Autodesk Inventor part; units mm, degrees
ref_plane "YZ Plane" through (0, 0, 0) normal (1, 0, 0) x (0, 1, 0)
ref_plane "XZ Plane" through (0, 0, 0) normal (0, 1, 0) x (-1, 0, 0)
ref_plane "XY Plane" through (0, 0, 0) normal (0, 0, 1) x (1, 0, 0)
sketch "Sketch1" plane through (0, 0, 0) normal (0, 0, 1) x (1, 0, 0)
  line L0 (-50, 50) -> (50, 50)
  line L1 (50, 50) -> (50, -50)
  line L2 (50, -50) -> (-50, -50)
  line L3 (-50, -50) -> (-50, 50)
  line L4 (-92.7646, -8.503) -> (-89.7646, -8.503)
  line L5 (-89.7646, -8.503) -> (-89.7646, -11.753)
  line L6 (-89.7646, -11.753) -> (-92.7646, -11.753)
  line L7 (-92.7646, -11.753) -> (-92.7646, -8.503)
  line L8 (-92.7646, -21.6527) -> (-89.7646, -21.6527)
  line L9 (-89.7646, -21.6527) -> (-89.7646, -21.7527)
  line L10 (-89.7646, -21.7527) -> (-92.7646, -21.7527)
  line L11 (-92.7646, -21.7527) -> (-92.7646, -21.6527)
  line L12 (-50, 50) -> (-46.75, 50)
  line L13 (-46.75, 50) -> (-46.75, 36)
  line L14 (-46.75, 36) -> (-50, 36)
  line L15 (-50, 36) -> (-50, 50)
  line L16 (0, 50) -> (0, -50) construction
  line L17 (-50, 0) -> (50, 0) construction
  line L18 (50, 50) -> (46.75, 50)
  line L19 (46.75, 50) -> (46.75, 36)
  line L20 (46.75, 36) -> (50, 36)
  line L21 (50, 36) -> (50, 50)
  line L22 (-50, -50) -> (-46.75, -50)
  line L23 (-46.75, -50) -> (-46.75, -36)
  line L24 (-46.75, -36) -> (-50, -36)
  line L25 (-50, -36) -> (-50, -50)
  line L26 (46.75, -50) -> (46.75, -36)
  line L27 (46.75, -36) -> (50, -36)
  line L28 (50, -36) -> (50, -50)
  line L29 (50, -50) -> (46.75, -50)
  line L30 (-40, -50) -> (-10, -50)
  line L31 (-10, -50) -> (-10, -37)
  line L32 (-17, -30) -> (-33, -30)
  line L33 (-40, -37) -> (-40, -50)
  line L34 (40, -50) -> (10, -50)
  line L35 (10, -50) -> (10, -37)
  line L36 (17, -30) -> (33, -30)
  line L37 (40, -37) -> (40, -50)
  line L38 (-1.75, -50) -> (-5, -50)
  line L39 (-5, -50) -> (-5, -42)
  line L40 (-5, -42) -> (-1.75, -42)
  line L41 (-1.75, -42) -> (-1.75, -50)
  line L42 (1.75, -50) -> (5, -50)
  line L43 (5, -50) -> (5, -42)
  line L44 (5, -42) -> (1.75, -42)
  line L45 (1.75, -42) -> (1.75, -50)
  arc A0 (-33, -30) -> (-40, -37) centre (-33, -37) ccw
  arc A1 (-10, -37) -> (-17, -30) centre (-17, -37) ccw
  arc A2 (17, -30) -> (10, -37) centre (17, -37) ccw
  arc A3 (40, -37) -> (33, -30) centre (33, -37) ccw
  point P0 (0, 0)
  point P1 (-10, -30)
  point P2 (-40, -30)
  point P3 (10, -30)
  point P4 (40, -30)
  dimension "d0" = 100
  dimension "d2" = 100
  dimension "d3" = 3
  dimension "mat" = 3.25
  dimension "d5" = 3
  dimension "kerf" = 0.1
  dimension "d7" = 3.25
  dimension "d8" = 14
  dimension "d15" = 30
  dimension "d16" = 20
  dimension "d17" = 10
  dimension "d20" = 3.25
  dimension "d21" = 8
  dimension "d22" = 5
  dimension "d25" = 45
  dimension "d26" = 7
extrude "Extrusion2" add sketch "Sketch1" along normal blind 3.25 contours L0 L19 L20 L1 L27 L26 L2 L37 A3 L36 A2 L35 L43 L44 L45 L41 L40 L39 L31 A1 L32 A0 L33 L23 L24 L3 L14 L13 | L39 L40 L41 L2 | L45 L44 L43 L2
extrude "Extrusion3" cut sketch "Sketch1" along normal blind 3.25 contours L39 L40 L41 L2 | L45 L44 L43 L2
equation "\"d7\" = mat"
equation "\"d20\" = mat"
equation "\"d18\" = mat"
equation "\"d23\" = mat"
properties part number "body-back"
Read the model definition and answer for the solid it produces. Units are mm, in the model's axes. A direction names the side the tool comes from. Round coordinates to 2 decimals unless told otherwise and drop trailing zeros. Loops run counter-clockwise (first coordinate to the right, second up) from the corner with the lowest first, then second, coordinate; pieces in that order, holes last. Notation, with made-up numbers: (34, 38.5) - (87, 38.5) arc R15 cw to (87, 58.5) - close; hole circle Ø4 at (89, 89). An arc over 180 degrees is marked (long way). One line per question, with ' | ' between items. Start each with the question number.
Q1. Section C-C on y = 39.5 is taken. Give the vertices of the cut face in (x, z).
Q2. For a pull along X with two mould halves and no side action, classify faces 5 (the flat face through (48, -36, 2)), 6 (the flat face through (-40, -43, 2)), 7 (the flat face through (-46.75, 43, 2)) as +X half, -X half, draft (parallel to the pull), parting line (faces both ways), or undercut.
Q3. For faces 1 (the flat face through (3, -42, 2)), 2 (the flat face through (46.75, 43, 2)), 3 (the flat face through (-46.75, -43, 2)), 4 (the flat face through (-48, 36, 2)), determine the directions among +Z, -Z, +X, -X, +Y, -Y from which every point of the face is accessible in a straight line to the end or side of a thin tool.
Q4. Find the intervals of material crossed by L1, parallel to X at y = -34, z = 1.35; L2, parallel to X at y = -33, z = 2.15; L3, parallel to Y at x = 17.5, z = 0.4, in increasing order.
Q5. Section B-B on x = -20 is taken. Give the vertices of the cut face in (y, z), plus the area to 3 significant figures.
Q6. Flat-ended cylindrical pins translate along their axes: pin 1 (1.6 mm diameter, centred on x = 48.5, z = 1, fed in from +Y); pin 2 (1.6 mm diameter, centred on y = -46, z = 1, fed in from +X). Find the tip coordinate at first contact, or state that the pin passes through.
Established:
1) outline: (-46.75, 0) - (46.75, 0) - (46.75, 3.25) - (-46.75, 3.25) - close
2) face 5: draft | face 6: undercut | face 7: -X half
3) face 1: +Z, -Z, -Y | face 2: +Z, -Z, +X, +Y | face 3: +Z, -Z, -X, -Y | face 4: +Z, -Z, -X, +Y
4) L1: -50 to -39.32, -10.68 to 10.68, 39.32 to 50 | L2: -50 to -38.74, -11.26 to 11.26, 38.74 to 50 | L3: -30 to 50
5) outline: (-30, 0) - (50, 0) - (50, 3.25) - (-30, 3.25) - close | area: 260 mm²
6) pin 1: y = 36 | pin 2: x = 46.75
